from build123d import *

# Parameters (mm, degrees)
SKETCH1_W                        = 70
SKETCH1_H                        = 50
BOSS_EXTRUDE1_DEPTH              = 12
SKETCH4_R                        = 47
BOSS_EXTRUDE2_DEPTH              = 24
SKETCH2_R                        = 31.5
CUT_EXTRUDE1_DEPTH               = 6
CBORE_START                      = -6
CBORE_FOR_M6_SHCS1_OUTLINE_R     = 3.3
CBORE_FOR_M6_SHCS1_DEPTH         = 18
CBORE_START_2                    = 6
CBORE_FOR_M6_SHCS1_2_OUTLINE_R   = 5.5
CBORE_FOR_M6_SHCS1_2_OUTLINE_R_2 = 3.3
CBORE_FOR_M6_SHCS1_2_DEPTH       = 6
CUT_EXTRUDE6_DEPTH               = 68.542579163
CUT_EXTRUDE6_DEPTH_BACK          = 68.542579163
M5_CLEARANCE_HOLE2_D             = 5.5
F_6_0MM_PRESS_DOWEL_HOLE2_D      = 6
SKETCH22_R                       = 12.5
CUT_EXTRUDE7_DEPTH               = 71.668239144
CUT_EXTRUDE8_DEPTH               = 10
CUT_EXTRUDE9_DEPTH               = 71.668239144
CHAMFER2_SIZE                    = 1


# Read off the part's stored shape, not the designer's step: CBORE for M6 SHCS1
with BuildPart() as part:
    # Sketch1 → Boss-Extrude1 (new, symmetric)
    with BuildSketch(Plane.XY):
        Rectangle(SKETCH1_W, SKETCH1_H)
    extrude(amount=BOSS_EXTRUDE1_DEPTH, both=True)

    # Sketch4 → Boss-Extrude2 (add, through all)
    with BuildSketch(Plane(origin=(0, 0, -12), x_dir=(-1, 0, 0), z_dir=(0, 0, -1))):
        Circle(SKETCH4_R)
    extrude(amount=-BOSS_EXTRUDE2_DEPTH)

    # Sketch2 → Cut-Extrude1 (cut)
    with BuildSketch(Plane(origin=(0, 0, -12), x_dir=(-1, 0, 0), z_dir=(0, 0, -1))):
        Circle(SKETCH2_R)
    extrude(amount=-CUT_EXTRUDE1_DEPTH, mode=Mode.SUBTRACT)

    # CBORE for M6 SHCS1 outline → CBORE for M6 SHCS1 (cut)
    with BuildSketch(Plane.XY.offset(CBORE_START)):
        with Locations((-17.67766953, -17.67766953)):
            Circle(CBORE_FOR_M6_SHCS1_OUTLINE_R)
        with Locations((-17.67766953, 17.67766953)):
            Circle(CBORE_FOR_M6_SHCS1_OUTLINE_R)
        with Locations((17.67766953, 17.67766953)):
            Circle(CBORE_FOR_M6_SHCS1_OUTLINE_R)
        with Locations((17.67766953, -17.67766953)):
            Circle(CBORE_FOR_M6_SHCS1_OUTLINE_R)
    extrude(amount=CBORE_FOR_M6_SHCS1_DEPTH, mode=Mode.SUBTRACT)

    # CBORE for M6 SHCS1 2 outline → CBORE for M6 SHCS1 2 (cut)
    # profile 1 of 4: a face of its own
    with BuildSketch(Plane.XY.offset(CBORE_START_2)):
        with Locations((-17.67766953, -17.67766953)):
            Circle(CBORE_FOR_M6_SHCS1_2_OUTLINE_R)
        with Locations((-17.67766953, -17.67766953)):
            Circle(CBORE_FOR_M6_SHCS1_2_OUTLINE_R_2, mode=Mode.SUBTRACT)
    # profile 2 of 4: a face of its own
    with BuildSketch(Plane.XY.offset(CBORE_START_2)):
        with Locations((-17.67766953, 17.67766953)):
            Circle(CBORE_FOR_M6_SHCS1_2_OUTLINE_R)
        with Locations((-17.67766953, 17.67766953)):
            Circle(CBORE_FOR_M6_SHCS1_2_OUTLINE_R_2, mode=Mode.SUBTRACT)
    # profile 3 of 4: a face of its own
    with BuildSketch(Plane.XY.offset(CBORE_START_2)):
        with Locations((17.67766953, 17.67766953)):
            Circle(CBORE_FOR_M6_SHCS1_2_OUTLINE_R)
        with Locations((17.67766953, 17.67766953)):
            Circle(CBORE_FOR_M6_SHCS1_2_OUTLINE_R_2, mode=Mode.SUBTRACT)
    # profile 4 of 4: a face of its own
    with BuildSketch(Plane.XY.offset(CBORE_START_2)):
        with Locations((17.67766953, -17.67766953)):
            Circle(CBORE_FOR_M6_SHCS1_2_OUTLINE_R)
        with Locations((17.67766953, -17.67766953)):
            Circle(CBORE_FOR_M6_SHCS1_2_OUTLINE_R_2, mode=Mode.SUBTRACT)
    extrude(amount=CBORE_FOR_M6_SHCS1_2_DEPTH, mode=Mode.SUBTRACT)

    # Sketch17 → Cut-Extrude6 (cut, two sides: drawn at the far end of the back side and taken through both)
    with BuildSketch(Plane.XZ.offset(-CUT_EXTRUDE6_DEPTH_BACK)):
        with BuildLine():
            Line((10, 16), (10, 6))
            ThreePointArc((10, 6), (0, -4), (-10, 6))
            Line((-10, 6), (-10, 16))
            ThreePointArc((-10, 16), (0, 26), (10, 16))
        make_face()
    extrude(amount=CUT_EXTRUDE6_DEPTH + CUT_EXTRUDE6_DEPTH_BACK, mode=Mode.SUBTRACT)

    # M5 Clearance Hole2 (through all)
    with Locations(Plane.XY.offset(12)):
        with Locations((-30, 25), (-30, -25), (30, -25), (30, 25)):
            Hole(M5_CLEARANCE_HOLE2_D / 2)

    # Ø6.0mm Press Dowel Hole2 (through all)
    with Locations(Plane.XY.offset(12)):
        with Locations((0, -25)):
            Hole(F_6_0MM_PRESS_DOWEL_HOLE2_D / 2)

    # Sketch22 → Cut-Extrude7 (cut, through all)
    with BuildSketch(Plane(origin=(0, 0, -12), x_dir=(-1, 0, 0), z_dir=(0, 0, -1))):
        with Locations((-25, 0)):
            Circle(SKETCH22_R)
        with Locations((25, 0)):
            Circle(SKETCH22_R)
    extrude(amount=-CUT_EXTRUDE7_DEPTH, mode=Mode.SUBTRACT)

    # Sketch23 → Cut-Extrude8 (cut)
    with BuildSketch(Plane(origin=(0, 0, -12), x_dir=(-1, 0, 0), z_dir=(0, 0, -1))):
        Polygon((-27.690598923, 29), (-32.309401077, 29), (-34.618802154, 25), (-32.309401077, 21), (-27.690598923, 21), (-25.381197846, 25), align=None)
        Polygon((-32.309401077, -21), (-34.618802154, -25), (-32.309401077, -29), (-27.690598923, -29), (-25.381197846, -25), (-27.690598923, -21), align=None)
        Polygon((32.309401077, -21), (27.690598923, -21), (25.381197846, -25), (27.690598923, -29), (32.309401077, -29), (34.618802154, -25), align=None)
        Polygon((27.690598923, 29), (25.381197846, 25), (27.690598923, 21), (32.309401077, 21), (34.618802154, 25), (32.309401077, 29), align=None)
    extrude(amount=-CUT_EXTRUDE8_DEPTH, mode=Mode.SUBTRACT)

    # Sketch24 → Cut-Extrude9 (cut, through all)
    with BuildSketch(Plane.XY.offset(12)):
        with BuildLine():
            ThreePointArc((-20.06863224, -42.5), (-15.131468813, -44.497625235), (-10, -45.923850013))
            Line((-10, -45.923850013), (-10, -42.5))
            Line((-10, -42.5), (-20.06863224, -42.5))
        make_face()
        with BuildLine():
            Line((-10, -42.5), (-10, -45.923850013))
            ThreePointArc((-10, -45.923850013), (0, -47), (10, -45.923850013))
            Line((10, -45.923850013), (10, -42.5))
            Line((10, -42.5), (-10, -42.5))
        make_face()
        with BuildLine():
            Line((10, -42.5), (10, -45.923850013))
            ThreePointArc((10, -45.923850013), (15.131468813, -44.497625235), (20.06863224, -42.5))
            Line((20.06863224, -42.5), (10, -42.5))
        make_face()
        with BuildLine():
            Line((42.5, 20.06863224), (42.5, -20.06863224))
            ThreePointArc((42.5, -20.06863224), (47, 0), (42.5, 20.06863224))
        make_face()
        with BuildLine():
            Line((10, 45.923850013), (10, 42.5))
            Line((10, 42.5), (20.06863224, 42.5))
            ThreePointArc((20.06863224, 42.5), (15.131468813, 44.497625235), (10, 45.923850013))
        make_face()
        with BuildLine():
            Line((-10, 45.923850013), (-10, 42.5))
            Line((-10, 42.5), (10, 42.5))
            Line((10, 42.5), (10, 45.923850013))
            ThreePointArc((10, 45.923850013), (0, 47), (-10, 45.923850013))
        make_face()
        with BuildLine():
            Line((-20.06863224, 42.5), (-10, 42.5))
            Line((-10, 42.5), (-10, 45.923850013))
            ThreePointArc((-10, 45.923850013), (-15.131468813, 44.497625235), (-20.06863224, 42.5))
        make_face()
        with BuildLine():
            ThreePointArc((-42.5, 20.06863224), (-47, 0), (-42.5, -20.06863224))
            Line((-42.5, -20.06863224), (-42.5, 20.06863224))
        make_face()
    extrude(amount=-CUT_EXTRUDE9_DEPTH, mode=Mode.SUBTRACT)

    # Chamfer2
    chamfer2_edges = [part.edges().sort_by_distance(p)[0] for p in [
        (-33.234018716, 33.234018716, -12),
        (-33.234018716, -33.234018716, 12),
        (-33.234018716, 33.234018716, 12),
        (33.234018716, 33.234018716, -12),
        (33.234018716, -33.234018716, -12),
        (-33.234018716, -33.234018716, -12),
        (33.234018716, 33.234018716, 12),
        (33.234018716, -33.234018716, 12),
        (0, -42.5, -12),
        (15.03431612, -42.5, 12),
        (-15.03431612, -42.5, 12),
        (42.5, 0, 12),
        (42.5, 0, -12),
        (-15.03431612, 42.5, 12),
        (15.03431612, 42.5, 12),
        (0, 42.5, -12),
        (-42.5, 0, -12),
        (-42.5, 0, 12),
    ]]
    chamfer(chamfer2_edges, length=CHAMFER2_SIZE)


solid = part.part
For this review, take the finished solid that the model builds, in its own axes (mm). A direction names the side the tool comes from. Give positions to 0.01 mm unless a question says otherwise; leave off trailing zeros. Loops run counter-clockwise (first coordinate to the right, second up) from the corner with the lowest first, then second, coordinate; pieces in that order, holes last.
Item 1: Take a section at A-A, the plane z = 8.25. Give the number of separate pieces and of enclosed holes in the cut face, and give its area (3 significant figures).
Item 2: Draft analysis for pull direction X (two halves, no side actions). For faces 4 (the flat face through (30, 21, -7)), 5 (the cylindrical face through (33.073, 33.394, -0.154)), 6 (the conical face through (-32.48, -32.8, -11.84)), state which applies: +X half, -X half, draft (parallel to the pull), parting line (faces both ways), or undercut.
Item 3: Take a section at B-B, the plane x = 0.5. State the section outline as (y, z) points.
Item 4: For line 1 along Y through (x, z) = (27.5, 0); line 2 along Y through (x, z) = (32, 6); line 3 along Z through (x, y) = (-20, 13), list the stretches that pass through material, from the lowest coordinate up.
Item 5: Take a section at C-C, the plane y = -4. State the section outline as (x, z) points, and give its area (3 significant figures).
Item 6: Insertion check: pin 1 (4 mm diameter, centred on y = -32, z = 1.5, fed in from -X); pin 2 (1.4 mm diameter, centred on x = 30, z = -6.5, fed in from +Y); pin 3 (9 mm diameter, centred on x = -30, y = -25, fed in from -Z); pin 4 (1 mm diameter, centred on x = 15.5, y = 26.5, fed in from -Z). Each pin has a flat end and moves straight along its axis. Give the tip position at first contact, or say it passes through.
Item 7: Tool access review of faces 1 (the flat face through (-30, 21, -7)), 2 (the cylindrical face through (20.63, 22.32, 8.96)), 3 (the cylindrical face through (16.962, 14.456, -0.084)): name each direction out of +Z, -Z, +X, -X, +Y, -Y from which nothing blocks a thin tool from reaching the whole face with its end or side.
Calculated:
1. separate pieces: 2
1. enclosed holes: 10
1. area: 3,300 mm2
2. face 4: undercut
2. face 5: +X half
2. face 6: -X half
3. outline: (-42.5, -11) - (-41.5, -12) - (-31.5, -12) - (-31.5, -6) - (-27.96, -6) - (-27.96, -3.99) - (-42.5, -3.99) - close; (-22.04, -6) - (31.5, -6) - (31.5, -12) - (41.5, -12) - (42.5, -11) - (42.5, -3.99) - (-22.04, -3.99) - close
4. line 1: y = -38.11 to -26.15, -23.85 to -12.25, 12.25 to 23.85, 26.15 to 38.11
4. line 2: y = -34.42 to -26.89, -23.11 to -10.36, 10.36 to 23.11, 26.89 to 34.42
4. line 3: z = -6 to 6
5. outline: (-42.5, -11) - (-41.5, -12) - (-36.84, -12) - (-36.84, 12) - (-41.5, 12) - (-42.5, 11) - close; (-13.16, -6) - (13.16, -6) - (13.16, 12) - (10, 12) - (10, 6) arc R10 cw to (-10, 6) - (-10, 12) - (-13.16, 12) - close; (36.84, -12) - (41.5, -12) - (42.5, -11) - (42.5, 11) - (41.5, 12) - (36.84, 12) - close
5. area: 466 mm2
6. pin 1: stops at x = -36.18
6. pin 2: stops at y = 36.75
6. pin 3: stops at z = -12
6. pin 4: stops at z = -6
7. face 1: -Z
7. face 2: +Z
7. face 3: +Z, -Z
